Job drawing, mm, ordinate dimensions from the low corner. One solid piece. A direction names the side the tool comes from. Round coordinates to 2 decimals unless told otherwise and drop trailing zeros. Loops run counter-clockwise (first coordinate to the right, second up) from the corner with the lowest first, then second, coordinate; pieces in that order, holes last. Notation, with made-up numbers: M 33,70.25 L 56,70.25 A15 ccw 56,81.25 Z; hole C -36,-33 d11. An arc over 180 degrees is marked long. Use a Markdown table: item, result. Add a question column.
(1) Band-saw the part on C-C, the plane z = 345. Write the cut outline in (x, y).
(2) Band-saw the part on D-D, the plane x = 465.5. Write the cut outline in (y, z), and give its area (3 significant figures).
(3) Band-saw the part on B-B, the plane y = 459.5. Write the cut outline in (x, z), and give its area (3 significant figures).
(4) Which spindle directions (+Z, -Z, +X, -X, +Y, -Y) get a long thin tool onto all of the face, cutting with end or side? Do the marked faces 1, 2, 3, 4 and 5. Say none if no direction does.
(5) Wall check: L1, parallel to Z at x = 591, y = 253.5; L2, parallel to X at y = 150, z = 227.5; L3, parallel to X at y = 248.5, z = 750.5. Give the ranges that are in metal, low to high.
(6) Band-saw the part on A-A, the plane x = 720. Write the cut outline in (y, z), and give its area (3 significant figures).
(7) Two-plate mould, pull along X, no slides. Class the marked faces 6, 7 and 8: released by +X, released by -X, zero draft, split by the parting line, or undercut.
(8) Flat gauge pin, fed straight in: P1, Ø10, axis at x = 726.5, z = 164.5, coming from the -Y side. Where does the tip first touch, or does it go through?
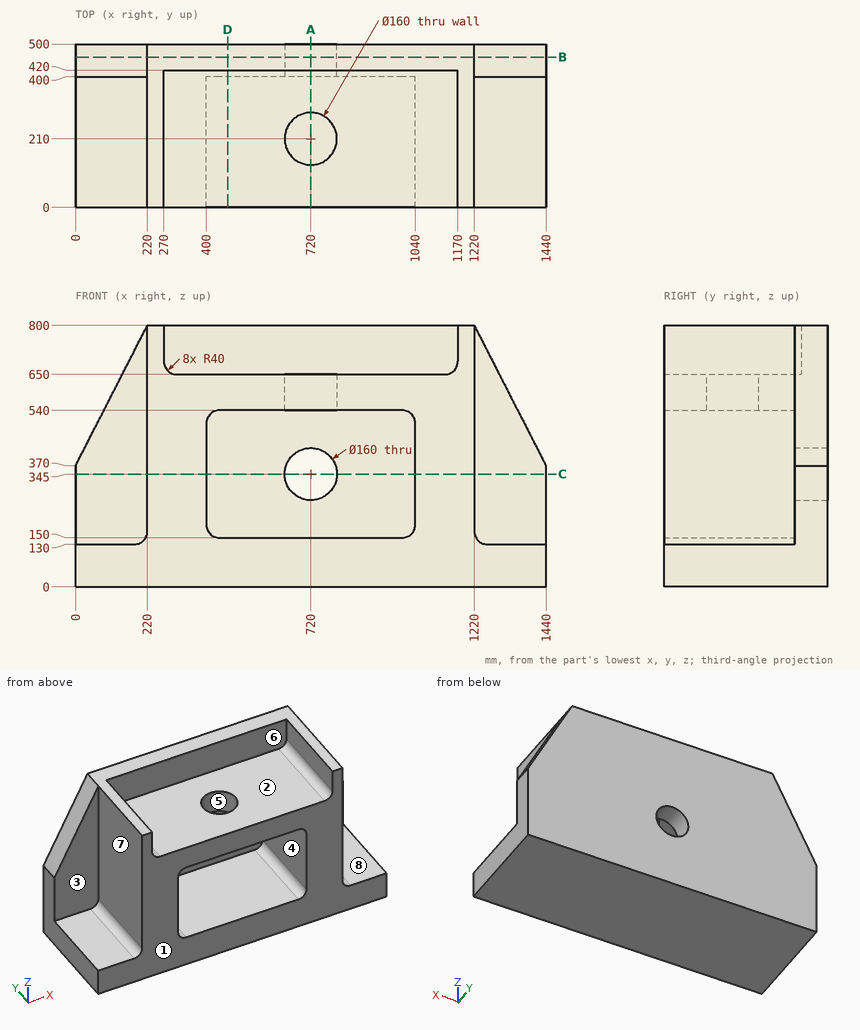
Return value:
| question | item | result |
|---|---|---|
| 1 | outline | M 0,400 L 220,400 L 220,0 L 400,0 L 400,400 L 640,400 L 640,500 L 0,500 Z; M 800,400 L 1040,400 L 1040,0 L 1220,0 L 1220,400 L 1440,400 L 1440,500 L 800,500 Z |
| 2 | outline | M 0,0 L 500,0 L 500,800 L 420,800 L 420,650 L 0,650 L 0,540 L 400,540 L 400,150 L 0,150 Z |
| 2 | area | 181,000 mm^2 |
| 3 | outline | M 0,0 L 1440,0 L 1440,370 L 1220,800 L 220,800 L 0,370 Z; hole C 720,345 d160 |
| 3 | area | 1,040,000 mm^2 |
| 4 | face 1 | +Z, -Z, +X, -X, -Y |
| 4 | face 2 | +Z, -Y |
| 4 | face 3 | +Z, -X, -Y |
| 4 | face 4 | -Y |
| 4 | face 5 | +Z |
| 5 | L1 | 0 to 150, 540 to 650 |
| 5 | L2 | 220 to 400, 1040 to 1220 |
| 5 | L3 | 220 to 270, 1170 to 1220 |
| 6 | outline | M 0,0 L 500,0 L 500,265 L 400,265 L 400,150 L 0,150 Z; M 0,540 L 130,540 L 130,650 L 0,650 Z; M 290,540 L 400,540 L 400,425 L 500,425 L 500,800 L 420,800 L 420,650 L 290,650 Z |
| 6 | area | 147,000 mm^2 |
| 7 | face 6 | undercut |
| 7 | face 7 | released by -X |
| 7 | face 8 | zero draft |
| 8 | P1 | y = 400 |
